Could you check a few things on this drawing? It's one solid part, dimensions in mm from its lowest x, y, z. A direction names the side the tool comes from. Give positions to 0.01 mm unless a question says otherwise; leave off trailing zeros. Write each loop counter-clockwise with the first axis right and the second up, starting at its lowest first coordinate (ties: lowest second). Pieces come first, ordered by that corner, then holes. Notation, with made-up numbers: M 74,-37.75 L 113,-37.75 A8 cw 113,-28.75 Z; hole C 42.25,69 d4. An arc over 180 degrees is marked long. Write each question's results on one line, items separated by ' | '.
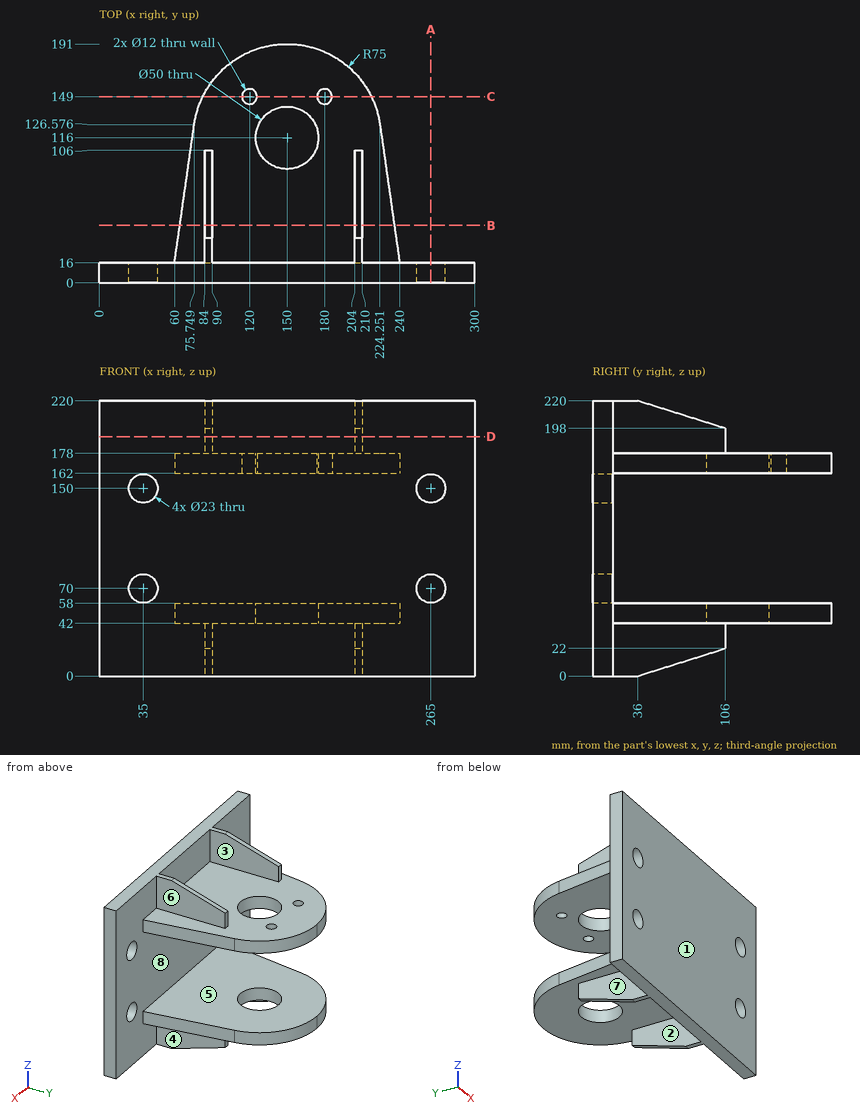
Item 1: I want a section at C-C, the plane y = 149. Please give me the cut outline in (x, z).
Geometry says:
outline: M 82.65,42 L 217.35,42 L 217.35,58 L 82.65,58 Z; M 82.65,162 L 114,162 L 114,178 L 82.65,178 Z; M 126,162 L 174,162 L 174,178 L 126,178 Z; M 186,162 L 217.35,162 L 217.35,178 L 186,178 Z
Item 2: Thinking about a two-plate mould opening in X: for the marked faces 1, 2, 3 and 4, which applies, +X half, -X half, draft (parallel to the pull), parting line (faces both ways), or undercut?
Geometry says:
face 1: draft | face 2: undercut | face 3: undercut | face 4: +X half
Item 3: If I drill on line 1 (X direction, y = 7, z = 70); line 2 (X direction, y = 31, z = 31); line 3 (Z direction, x = 160, y = 175.5), over which ranges is the centre line in solid material (lowest first)? Write a range as from..to.
Geometry says:
line 1: x = 0..23.5, 46.5..253.5, 276.5..300 | line 2: x = 84..90, 204..210 | line 3: z = 42..58, 162..178
Item 4: I want a section at B-B, the plane y = 46. Please give me the cut outline in (x, z).
Geometry says:
outline: M 64.27,42 L 84,42 L 84,3.14 L 90,3.14 L 90,42 L 204,42 L 204,3.14 L 210,3.14 L 210,42 L 235.73,42 L 235.73,58 L 64.27,58 Z; M 64.27,162 L 235.73,162 L 235.73,178 L 210,178 L 210,216.86 L 204,216.86 L 204,178 L 90,178 L 90,216.86 L 84,216.86 L 84,178 L 64.27,178 Z
Item 5: I want a section at D-D, the plane z = 191.5. Please give me the cut outline in (x, y).
Geometry says:
outline: M 0,0 L 300,0 L 300,16 L 210,16 L 210,106 L 204,106 L 204,16 L 90,16 L 90,106 L 84,106 L 84,16 L 0,16 Z
Item 6: I'm going to push flat-ended pins straight in: pin 1 (12 mm diameter, centred on x = 176, y = 150.5, fed in from +Z); pin 2 (19 mm diameter, centred on x = 120, y = 149, fed in from -Z); pin 3 (2 mm diameter, centred on y = 84.5, z = 27.5, fed in from +X); pin 4 (3 mm diameter, centred on x = 212, z = 192.5, fed in from -Y). Where does each tip first touch, or does it pass through?
Geometry says:
pin 1: stops at z = 178 | pin 2: stops at z = 42 | pin 3: stops at x = 210 | pin 4: stops at y = 0
Item 7: I want a section at A-A, the plane x = 265. Please give me the cut outline in (y, z).
Geometry says:
outline: M 0,0 L 16,0 L 16,58.5 L 0,58.5 Z; M 0,81.5 L 16,81.5 L 16,138.5 L 0,138.5 Z; M 0,161.5 L 16,161.5 L 16,220 L 0,220 Z
Item 8: For the marked faces 5, 6, 7 and 8, which set-ups out of +Z, -Z, +X, -X, +Y, -Y let a thin tool reach every point of the face, with its end or its side?
Geometry says:
face 5: +X, -X, +Y | face 6: +Z, +X, +Y | face 7: -Z, -X, +Y | face 8: +Y
